Check sheet for the modelled part. Datum: model origin and axes. Units: mm. Face numbers are marked on the shaded views. A direction names the side the tool comes from. Round coordinates to 2 decimals unless told otherwise and drop trailing zeros. Write each loop counter-clockwise with the first axis right and the second up, starting at its lowest first coordinate (ties: lowest second). Pieces come first, ordered by that corner, then holes. Notation, with made-up numbers: M 21,32.25 L 54,32.25 A22 ccw 54,60.25 Z; hole C 35,15 d9. An arc over 180 degrees is marked long. Put each result on its own line as item: value.
```python
from build123d import *

# Parameters (mm, degrees)
CROQUIS1_W              = 190
CROQUIS1_H              = 190
SALIENTE_EXTRUIR1_DEPTH = 45
VACIADO1_T              = -3
CROQUIS4_W              = 60
CROQUIS4_H              = 30
CORTAR_EXTRUIR1_DEPTH   = 226.78881097
CROQUIS7_W              = 190
CROQUIS7_H              = 45
CORTAR_EXTRUIR2_DEPTH   = 3


with BuildPart() as part:
    # Croquis1 → Saliente-Extruir1 (new body)
    with BuildSketch(Plane.XY):
        with Locations((56.932555838, -65.848020305)):
            Rectangle(CROQUIS1_W, CROQUIS1_H)
    extrude(amount=-SALIENTE_EXTRUIR1_DEPTH)

    # Vaciado1
    vaciado1_openings = [part.faces().sort_by_distance(p)[0] for p in [
        (56.932555838, -65.848020305, -45),
    ]]
    offset(amount=VACIADO1_T, openings=vaciado1_openings, kind=Kind.INTERSECTION)

    # Croquis4 → Cortar-Extruir1 (cut, through all)
    with BuildSketch(Plane.XY):
        with Locations((-8.067444162, -145.848020305)):
            Rectangle(CROQUIS4_W, CROQUIS4_H)
    extrude(amount=-CORTAR_EXTRUIR1_DEPTH, mode=Mode.SUBTRACT)

    # Croquis7 → Cortar-Extruir2 (cut)
    with BuildSketch(Plane(origin=(0, 29.151979695, 0), x_dir=(1, 0, 0), z_dir=(0, 1, 0))):
        with Locations((56.932555838, 22.5)):
            Rectangle(CROQUIS7_W, CROQUIS7_H)
    extrude(amount=-CORTAR_EXTRUIR2_DEPTH, mode=Mode.SUBTRACT)


solid = part.part
```
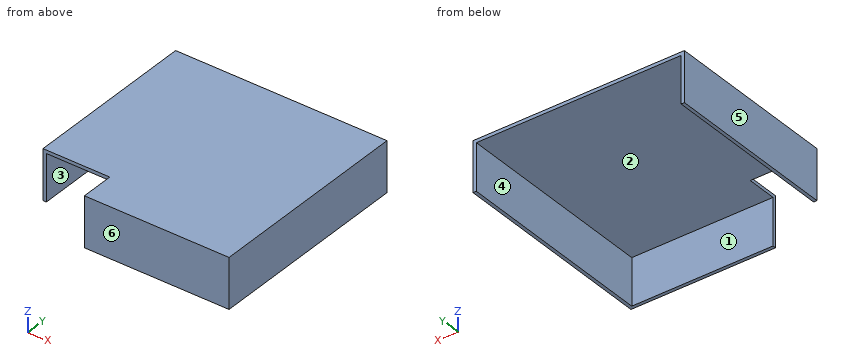
1. Depth check by flat-ended pin: pin 1 Ø12 at (x, y) = (-11.5, -28) entering from -Z; pin 2 Ø2 at (x, z) = (39, -10.5) entering from +Y; pin 3 Ø15 at (y, z) = (-145, -20.5) entering from -X. Enter the tip coordinate at first touch or a pass-through.
Computed values:
pin 1: stops at z = -3
pin 2: stops at y = -157.85
pin 3: stops at x = 148.93
2. Cross-section at D-D (y = -147). Enter the section's corners in (x, z), then the cut area to 3 significant figures.
Computed values:
outline: M 21.93,-3 L 148.93,-3 L 148.93,-45 L 151.93,-45 L 151.93,0 L 21.93,0 Z
area: 516 mm2
3. Cross-section at B-B (y = -30). Enter the section's corners in (x, z).
Computed values:
outline: M -38.07,-45 L -35.07,-45 L -35.07,-3 L 148.93,-3 L 148.93,-45 L 151.93,-45 L 151.93,0 L -38.07,0 Z
4. Cross-section at C-C (x = 119.5). Enter the section's corners in (y, z).
Computed values:
outline: M -160.85,-45 L -157.85,-45 L -157.85,-3 L 26.15,-3 L 26.15,0 L -160.85,0 Z
5. Release check for a two-part mould opening along X. For the marked faces 4, 5 and 6 record: +X half, -X half, draft (parallel to the pull), parting line (faces both ways), or undercut.
Computed values:
face 4: undercut
face 5: -X half
face 6: draft
6. Access from +Z, -Z, +X, -X, +Y, -Y to the whole of each face (thin tool, end or side, straight path). Record for the marked faces 1, 2 and 3.
Computed values:
face 1: -Z, -X, +Y
face 2: -Z, +Y
face 3: -Z, +Y, -Y
7. Cross-section at A-A (z = -9). Enter the section's corners in (x, y), then the cut area to 3 significant figures.
Computed values:
outline: M -38.07,-130.85 L -35.07,-130.85 L -35.07,26.15 L -38.07,26.15 Z; M 21.93,-160.85 L 151.93,-160.85 L 151.93,26.15 L 148.93,26.15 L 148.93,-157.85 L 21.93,-157.85 Z
area: 1,410 mm2
8. Scan lines: probe 1 along X at (y, z) = (-85, -39); probe 2 along Z at (x, y) = (56, -56); probe 3 along Y at (x, z) = (118.5, -16). Record each from-to range of solid material in increasing order.
Computed values:
probe 1: x = -38.07 to -35.07, 148.93 to 151.93
probe 2: z = -3 to 0
probe 3: y = -160.85 to -157.85
